from build123d import *

# Parameters (mm, degrees)
SKETCH1_W           = 53.8
SKETCH1_H           = 40
SKETCH1_R           = 2.1
SKETCH1_R_2         = 4
BOSS_EXTRUDE1_DEPTH = 10
SKETCH2_R           = 11
CUT_EXTRUDE1_DEPTH  = 7.5
SKETCH3_W           = 53.8
SKETCH3_H           = 10
CUT_EXTRUDE2_DEPTH  = 2
SKETCH4_W           = 53.8
SKETCH4_H           = 10
CUT_EXTRUDE3_DEPTH  = 2


with BuildPart() as part:
    # Sketch1 → Boss-Extrude1 (new body)
    with BuildSketch(Plane.XY):
        with Locations((-26.9, 20)):
            Rectangle(SKETCH1_W, SKETCH1_H)
        with Locations((-22.5, 32.5)):
            Circle(SKETCH1_R, mode=Mode.SUBTRACT)
        with Locations((-47.5, 7.5)):
            Circle(SKETCH1_R, mode=Mode.SUBTRACT)
        with Locations((-47.5, 32.5)):
            Circle(SKETCH1_R, mode=Mode.SUBTRACT)
        with Locations((-22.5, 7.5)):
            Circle(SKETCH1_R, mode=Mode.SUBTRACT)
        with Locations((-5, 32.5)):
            Circle(SKETCH1_R, mode=Mode.SUBTRACT)
        with Locations((-5, 7.5)):
            Circle(SKETCH1_R, mode=Mode.SUBTRACT)
        with Locations((-35, 20)):
            Circle(SKETCH1_R_2, mode=Mode.SUBTRACT)
    extrude(amount=BOSS_EXTRUDE1_DEPTH)

    # Sketch2 → Cut-Extrude1 (cut)
    with BuildSketch(Plane(origin=(0, 0, 0), x_dir=(-1, 0, 0), z_dir=(0, 0, -1))):
        with Locations((35, 20)):
            Circle(SKETCH2_R)
    extrude(amount=-CUT_EXTRUDE1_DEPTH, mode=Mode.SUBTRACT)

    # Sketch3 → Cut-Extrude2 (cut)
    with BuildSketch(Plane.XZ):
        with Locations((-26.9, 5)):
            Rectangle(SKETCH3_W, SKETCH3_H)
    extrude(amount=-CUT_EXTRUDE2_DEPTH, mode=Mode.SUBTRACT)

    # Sketch4 → Cut-Extrude3 (cut)
    with BuildSketch(Plane(origin=(0, 40, 0), x_dir=(1, 0, 0), z_dir=(0, 1, 0))):
        with Locations((-26.9, -5)):
            Rectangle(SKETCH4_W, SKETCH4_H)
    extrude(amount=-CUT_EXTRUDE3_DEPTH, mode=Mode.SUBTRACT)


solid = part.part
Part model, mm, in its own coordinate system. A direction names the side the tool comes from. Give positions to 0.01 mm unless a question says otherwise; leave off trailing zeros. Loops run counter-clockwise (first coordinate to the right, second up) from the corner with the lowest first, then second, coordinate; pieces in that order, holes last. Notation, with made-up numbers: M 73.25,51.5 L 129.25,51.5 A18 cw 129.25,67.5 Z; hole C -1,49.5 d6. An arc over 180 degrees is marked long. Put each result on its own line as item: value. Start each with the question number.
1) Saw through at B-B (y = 32.5). List the corners of the cut face in (x, z).
2) Saw through at D-D (y = 20). List the corners of the cut face in (x, z), then the cut area to 3 significant figures.
3) Probe probe 1 along Y at (x, z) = (-47.5, 3.5); probe 2 along X at (y, z) = (20, 8.9); probe 3 along Y at (x, z) = (-35, 3.25). List the from-to ranges inside material, lowest first.
4) Saw through at C-C (z = 8.25). List the corners of the cut face in (x, y), then the cut area to 3 significant figures.
5) 3-axis set-ups, long thin cutter, end or side, ignore diameter. For faces 1 (the flat face through (-35, 15, 7.5)), 2 (the flat face through (-21, 20, 0)): which of +Z, -Z, +X, -X, +Y, -Y reach the whole face in a straight line?
6) Flat gauge pin, fed straight in: pin 1 (11 mm diameter, centred on x = -31.5, y = 20, fed in from -Z). Where does the tip first touch, or does it go through?
7) Saw through at A-A (x = -5). List the corners of the cut face in (y, z), then the cut area to 3 significant figures.
8) Pull direction X, two halves, no side cores. Call faces 3 (the flat face through (-53.8, 20, 5)), 4 (the flat face through (0, 20, 5)), 5 (the cylindrical face through (-46.531, 30.637, 4.93)): +X half, -X half, draft (parallel to the pull), parting line (faces both ways), or undercut.
Numbers:
1. outline: M -53.8,0 L -49.6,0 L -49.6,10 L -53.8,10 Z; M -45.4,0 L -24.6,0 L -24.6,10 L -45.4,10 Z; M -20.4,0 L -7.1,0 L -7.1,10 L -20.4,10 Z; M -2.9,0 L 0,0 L 0,10 L -2.9,10 Z
2. outline: M -53.8,0 L -46,0 L -46,7.5 L -39,7.5 L -39,10 L -53.8,10 Z; M -31,7.5 L -24,7.5 L -24,0 L 0,0 L 0,10 L -31,10 Z
2. area: 353 mm^2
3. probe 1: 2 to 5.4, 9.6 to 30.4, 34.6 to 38
3. probe 2: -53.8 to -39, -31 to 0
3. probe 3: 2 to 9, 31 to 38
4. outline: M -53.8,2 L 0,2 L 0,38 L -53.8,38 Z; hole C -47.5,7.5 d4.2; hole C -47.5,32.5 d4.2; hole C -35,20 d8; hole C -22.5,7.5 d4.2; hole C -22.5,32.5 d4.2; hole C -5,7.5 d4.2; hole C -5,32.5 d4.2
4. area: 1,800 mm^2
5. face 1: -Z
5. face 2: -Z, +X, -X, +Y, -Y
6. pin 1: z = 7.5
7. outline: M 2,0 L 5.4,0 L 5.4,10 L 2,10 Z; M 9.6,0 L 30.4,0 L 30.4,10 L 9.6,10 Z; M 34.6,0 L 38,0 L 38,10 L 34.6,10 Z
7. area: 276 mm^2
8. face 3: -X half
8. face 4: +X half
8. face 5: undercut
